from build123d import *

# Parameters (mm, degrees)
SKETCH1_R           = 16.5
BOSS_EXTRUDE1_DEPTH = 22
SKETCH2_W           = 2.99551857
SKETCH2_H           = 2.853303302
SKETCH2_W_2         = 2.853303302
SKETCH2_H_2         = 2.99551857
CUT_EXTRUDE1_DEPTH  = 2.5
SKETCH3_R           = 4
BOSS_EXTRUDE2_DEPTH = 2.2
CUT_EXTRUDE2_DEPTH  = 12.2
SKETCH5_W           = 3.219111416
SKETCH5_H           = 1.024262723
BOSS_EXTRUDE3_DEPTH = 3
CUT_EXTRUDE3_DEPTH  = 3
CIRPATTERN2_COUNT   = 2
SHELL1_START        = 2
SHELL1_DEPTH        = 20
SHELL1_START_2      = 14.2
SHELL1_2_DEPTH      = 7.8
SHELL1_START_3      = 4.5
SHELL1_3_DEPTH      = 9.7
SHELL1_START_4      = -0.2
SHELL1_4_OUTLINE_R  = 2
SHELL1_4_DEPTH      = 2.2
SKETCH7_R           = 9.780494134
CUT_EXTRUDE4_DEPTH  = 28
SKETCH8_R           = 16.5
SKETCH8_R_2         = 16.427034369
CUT_EXTRUDE5_DEPTH  = 0.3
FILLET1_R           = 0.3
FILLET2_R           = 0.8
SKETCH9_W           = 19.2
SKETCH9_H           = 1.567367832
SKETCH9_H_2         = 1.325546631
BOSS_EXTRUDE4_DEPTH = 3


# Read off the part's stored shape, not the designer's step: Shell1
with BuildPart() as part:
    # Sketch1 → Boss-Extrude1 (new body)
    with BuildSketch(Plane(origin=(0, 0, 0), x_dir=(0, 0, -1), z_dir=(1, 0, 0))):
        Circle(SKETCH1_R)
    extrude(amount=BOSS_EXTRUDE1_DEPTH)

    # Sketch2 → Cut-Extrude1 (cut)
    with BuildSketch(Plane.ZY):
        with Locations((-16.5, 0)):
            Rectangle(SKETCH2_W, SKETCH2_H)
        with Locations((0, 16.5)):
            Rectangle(SKETCH2_W_2, SKETCH2_H_2)
        with Locations((16.5, 0)):
            Rectangle(SKETCH2_W, SKETCH2_H)
        with Locations((0, -16.5)):
            Rectangle(SKETCH2_W_2, SKETCH2_H_2)
    extrude(amount=-CUT_EXTRUDE1_DEPTH, mode=Mode.SUBTRACT)

    # Sketch3 → Boss-Extrude2 (add)
    with BuildSketch(Plane.ZY):
        Circle(SKETCH3_R)
    extrude(amount=BOSS_EXTRUDE2_DEPTH)

    # Sketch4 → Cut-Extrude2 (cut)
    with BuildSketch(Plane.ZY):
        with BuildLine():
            ThreePointArc((2.706980055, 5.596864168), (0.036580812, 6.702979752), (-2.633818432, 5.596864168))
            ThreePointArc((-2.633818432, 5.596864168), (-2.633818432, 4.865247937), (-1.902202201, 4.865247937))
            ThreePointArc((-1.902202201, 4.865247937), (0.036580812, 5.668318155), (1.975363824, 4.865247937))
            ThreePointArc((1.975363824, 4.865247937), (2.706980055, 4.865247937), (2.706980055, 5.596864168))
        make_face()
        with BuildLine():
            ThreePointArc((-2.706980055, -5.596864168), (-0.036580812, -6.702979752), (2.633818432, -5.596864168))
            ThreePointArc((2.633818432, -5.596864168), (2.633818432, -4.865247937), (1.902202201, -4.865247937))
            ThreePointArc((1.902202201, -4.865247937), (-0.036580812, -5.668318155), (-1.975363824, -4.865247937))
            ThreePointArc((-1.975363824, -4.865247937), (-2.706980055, -4.865247937), (-2.706980055, -5.596864168))
        make_face()
    extrude(amount=-CUT_EXTRUDE2_DEPTH, mode=Mode.SUBTRACT)

    # Sketch5 → Boss-Extrude3 (add)
    with BuildSketch(Plane.ZY):
        with Locations((0, 11.230309148)):
            Rectangle(SKETCH5_W, SKETCH5_H)
    boss_extrude3 = extrude(amount=BOSS_EXTRUDE3_DEPTH)

    # Sketch6 → Cut-Extrude3 (cut)
    with BuildSketch(Plane(origin=(0, 11.742440509, 0), x_dir=(1, 0, 0), z_dir=(0, 1, 0))):
        with BuildLine():
            Line((-1.239883538, -0.443858464), (-2.275602474, -0.443858464))
            ThreePointArc((-2.275602474, -0.443858464), (-2.719460937, 0), (-2.275602474, 0.443858464))
            Line((-2.275602474, 0.443858464), (-1.239883538, 0.443858464))
            ThreePointArc((-1.239883538, 0.443858464), (-0.796025074, 0), (-1.239883538, -0.443858464))
        make_face()
    cut_extrude3 = extrude(amount=-CUT_EXTRUDE3_DEPTH, mode=Mode.SUBTRACT)

    # CirPattern2: Boss-Extrude3, Cut-Extrude3 ×2 about axis
    cirpattern2_axis = Axis((0, 0, 0), (1, 0, 0))
    add([boss_extrude3.rotate(cirpattern2_axis, i * 360 / CIRPATTERN2_COUNT) for i in range(1, CIRPATTERN2_COUNT)])
    add([cut_extrude3.rotate(cirpattern2_axis, i * 360 / CIRPATTERN2_COUNT) for i in range(1, CIRPATTERN2_COUNT)], mode=Mode.SUBTRACT)

    # Shell1 outline → Shell1 (cut)
    with BuildSketch(Plane.YZ.offset(SHELL1_START)):
        with BuildLine():
            Line((13.002240715, 3.426651651), (14.089288785, 3.426651651))
            ThreePointArc((14.089288785, 3.426651651), (10.253048327, 10.253048327), (3.426651651, 14.089288785))
            Line((3.426651651, 14.089288785), (3.426651651, 13.002240715))
            Line((3.426651651, 13.002240715), (-3.426651651, 13.002240715))
            Line((-3.426651651, 13.002240715), (-3.426651651, 14.089288785))
            ThreePointArc((-3.426651651, 14.089288785), (-10.253048327, 10.253048327), (-14.089288785, 3.426651651))
            Line((-14.089288785, 3.426651651), (-13.002240715, 3.426651651))
            Line((-13.002240715, 3.426651651), (-13.002240715, -3.426651651))
            Line((-13.002240715, -3.426651651), (-14.089288785, -3.426651651))
            ThreePointArc((-14.089288785, -3.426651651), (-10.253048327, -10.253048327), (-3.426651651, -14.089288785))
            Line((-3.426651651, -14.089288785), (-3.426651651, -13.002240715))
            Line((-3.426651651, -13.002240715), (3.426651651, -13.002240715))
            Line((3.426651651, -13.002240715), (3.426651651, -14.089288785))
            ThreePointArc((3.426651651, -14.089288785), (10.253048327, -10.253048327), (14.089288785, -3.426651651))
            Line((14.089288785, -3.426651651), (13.002240715, -3.426651651))
            Line((13.002240715, -3.426651651), (13.002240715, 3.426651651))
        make_face()
        with BuildLine():
            ThreePointArc((-3.451034375, 0.487988639), (-3.668318155, -0.036580811), (-3.451034375, -0.561150262))
            ThreePointArc((-3.451034375, -0.561150262), (-3.451034375, -4.121193617), (-7.01107773, -4.121193617))
            ThreePointArc((-7.01107773, -4.121193617), (-8.702979752, -0.036580811), (-7.01107773, 4.048031994))
            ThreePointArc((-7.01107773, 4.048031994), (-3.451034375, 4.048031994), (-3.451034375, 0.487988639))
        make_face(mode=Mode.SUBTRACT)
        with BuildLine():
            ThreePointArc((3.451034375, -0.487988639), (3.668318155, 0.036580811), (3.451034375, 0.561150262))
            ThreePointArc((3.451034375, 0.561150262), (3.451034375, 4.121193617), (7.01107773, 4.121193617))
            ThreePointArc((7.01107773, 4.121193617), (8.702979752, 0.036580811), (7.01107773, -4.048031994))
            ThreePointArc((7.01107773, -4.048031994), (3.451034375, -4.048031994), (3.451034375, -0.487988639))
        make_face(mode=Mode.SUBTRACT)
    extrude(amount=SHELL1_DEPTH, mode=Mode.SUBTRACT)

    # Shell1 2 outline → Shell1 2 (cut)
    with BuildSketch(Plane.YZ.offset(SHELL1_START_2)):
        with BuildLine():
            ThreePointArc((14.089288785, -3.426651651), (14.5, 0), (14.089288785, 3.426651651))
            Line((14.089288785, 3.426651651), (13.002240715, 3.426651651))
            Line((13.002240715, 3.426651651), (13.002240715, -3.426651651))
            Line((13.002240715, -3.426651651), (14.089288785, -3.426651651))
        make_face()
        with BuildLine():
            Line((3.426651651, 13.002240715), (3.426651651, 14.089288785))
            ThreePointArc((3.426651651, 14.089288785), (0, 14.5), (-3.426651651, 14.089288785))
            Line((-3.426651651, 14.089288785), (-3.426651651, 13.002240715))
            Line((-3.426651651, 13.002240715), (3.426651651, 13.002240715))
        make_face()
        with BuildLine():
            ThreePointArc((-3.426651651, -14.089288785), (0, -14.5), (3.426651651, -14.089288785))
            Line((3.426651651, -14.089288785), (3.426651651, -13.002240715))
            Line((3.426651651, -13.002240715), (-3.426651651, -13.002240715))
            Line((-3.426651651, -13.002240715), (-3.426651651, -14.089288785))
        make_face()
        with BuildLine():
            Line((-13.002240715, 3.426651651), (-14.089288785, 3.426651651))
            ThreePointArc((-14.089288785, 3.426651651), (-14.5, 0), (-14.089288785, -3.426651651))
            Line((-14.089288785, -3.426651651), (-13.002240715, -3.426651651))
            Line((-13.002240715, -3.426651651), (-13.002240715, 3.426651651))
        make_face()
        with BuildLine():
            ThreePointArc((-7.01107773, -4.121193617), (-3.451034375, -4.121193617), (-3.451034375, -0.561150262))
            ThreePointArc((-3.451034375, -0.561150262), (-3.668318155, -0.036580811), (-3.451034375, 0.487988639))
            ThreePointArc((-3.451034375, 0.487988639), (-3.451034375, 4.048031994), (-7.01107773, 4.048031994))
            ThreePointArc((-7.01107773, 4.048031994), (-8.702979752, -0.036580811), (-7.01107773, -4.121193617))
        make_face()
        with BuildLine():
            ThreePointArc((7.01107773, 4.121193617), (3.451034375, 4.121193617), (3.451034375, 0.561150262))
            ThreePointArc((3.451034375, 0.561150262), (3.668318155, 0.036580811), (3.451034375, -0.487988639))
            ThreePointArc((3.451034375, -0.487988639), (3.451034375, -4.048031994), (7.01107773, -4.048031994))
            ThreePointArc((7.01107773, -4.048031994), (8.702979752, 0.036580811), (7.01107773, 4.121193617))
        make_face()
    extrude(amount=SHELL1_2_DEPTH, mode=Mode.SUBTRACT)

    # Shell1 3 outline → Shell1 3 (cut)
    with BuildSketch(Plane.YZ.offset(SHELL1_START_3)):
        with BuildLine():
            ThreePointArc((14.089288785, -3.426651651), (14.5, 0), (14.089288785, 3.426651651))
            Line((14.089288785, 3.426651651), (13.002240715, 3.426651651))
            Line((13.002240715, 3.426651651), (13.002240715, -3.426651651))
            Line((13.002240715, -3.426651651), (14.089288785, -3.426651651))
        make_face()
        with BuildLine():
            Line((3.426651651, 13.002240715), (3.426651651, 14.089288785))
            ThreePointArc((3.426651651, 14.089288785), (0, 14.5), (-3.426651651, 14.089288785))
            Line((-3.426651651, 14.089288785), (-3.426651651, 13.002240715))
            Line((-3.426651651, 13.002240715), (3.426651651, 13.002240715))
        make_face()
        with BuildLine():
            ThreePointArc((-3.426651651, -14.089288785), (0, -14.5), (3.426651651, -14.089288785))
            Line((3.426651651, -14.089288785), (3.426651651, -13.002240715))
            Line((3.426651651, -13.002240715), (-3.426651651, -13.002240715))
            Line((-3.426651651, -13.002240715), (-3.426651651, -14.089288785))
        make_face()
        with BuildLine():
            Line((-13.002240715, 3.426651651), (-14.089288785, 3.426651651))
            ThreePointArc((-14.089288785, 3.426651651), (-14.5, 0), (-14.089288785, -3.426651651))
            Line((-14.089288785, -3.426651651), (-13.002240715, -3.426651651))
            Line((-13.002240715, -3.426651651), (-13.002240715, 3.426651651))
        make_face()
    extrude(amount=SHELL1_3_DEPTH, mode=Mode.SUBTRACT)

    # Shell1 4 outline → Shell1 4 (cut)
    with BuildSketch(Plane.YZ.offset(SHELL1_START_4)):
        Circle(SHELL1_4_OUTLINE_R)
    extrude(amount=SHELL1_4_DEPTH, mode=Mode.SUBTRACT)

    # Sketch7 → Cut-Extrude4 (cut)
    with BuildSketch(Plane(origin=(2, 0, 0), x_dir=(0, 0, -1), z_dir=(1, 0, 0))):
        Circle(SKETCH7_R)
    extrude(amount=CUT_EXTRUDE4_DEPTH, mode=Mode.SUBTRACT)

    # Sketch8 → Cut-Extrude5 (cut)
    with BuildSketch(Plane.ZY.offset(-2.5)):
        Circle(SKETCH8_R)
        Circle(SKETCH8_R_2, mode=Mode.SUBTRACT)
    extrude(amount=-CUT_EXTRUDE5_DEPTH, mode=Mode.SUBTRACT)

    # Fillet1
    fillet1_edges = [part.edges().sort_by_distance(p)[0] for p in [
        (0, 11.66726189, -11.66726189),
        (0, 11.66726189, 11.66726189),
        (0, -11.66726189, 11.66726189),
        (0, -11.66726189, -11.66726189),
    ]]
    fillet(fillet1_edges, radius=FILLET1_R)

    # Fillet2
    fillet2_edges = [part.edges().sort_by_distance(p)[0] for p in [
        (-3, 11.230309148, 1.609555708),
        (-3, 11.230309148, -1.609555708),
        (-3, -11.230309148, -1.609555708),
        (-3, -11.230309148, 1.609555708),
    ]]
    fillet(fillet2_edges, radius=FILLET2_R)

    # Sketch9 → Boss-Extrude4 (add)
    with BuildSketch(Plane.XY.offset(-14.58)):
        with Locations((12.4, 6.833683916)):
            Rectangle(SKETCH9_W, SKETCH9_H)
        with Locations((12.4, -6.712773316)):
            Rectangle(SKETCH9_W, SKETCH9_H_2)
    extrude(amount=-BOSS_EXTRUDE4_DEPTH)


solid = part.part
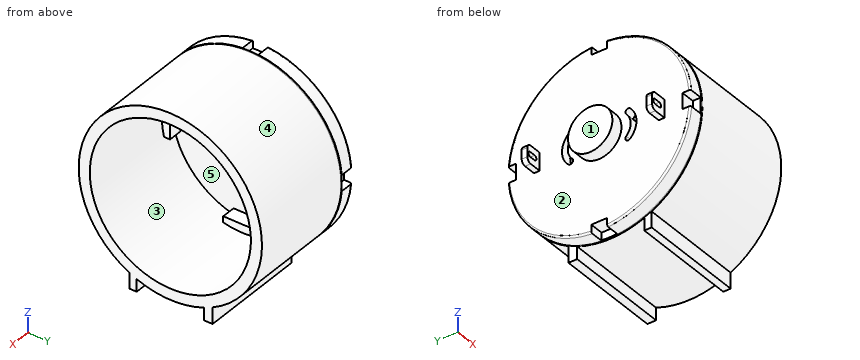
Geometry: final body of the model. Coordinates: model frame, mm. Face numbers are marked on the shaded views. A direction names the side the tool comes from. Round coordinates to 2 decimals unless told otherwise and drop trailing zeros. Order: outer loops, then holes, each group sorted by start corner. A loop starts at its lowest first (then second) coordinate and runs counter-clockwise, first axis right, second up.
Q1. Access query for the marked faces 1, 2 and 3. Directions: +Z, -Z, +X, -X, +Y, -Y. A direction counts if a zero-diameter tool reaches every point of the face in a straight line with its end or side. Return the directions, or none.
Result sheet:
face 1: +Z, -Z, -X
face 2: -X
face 3: +X
Q2. Pin query (flat end, axial travel): pin 1 (2 mm diameter, centred on x = 11, y = -4.5, fed in from -Z); pin 2 (0.8 mm diameter, centred on x = -1.5, y = 11.5, fed in from -Z); pin 3 (2 mm diameter, centred on y = 1, z = 0.5, fed in from +X). Return the tip coordinate at first contact, or that it passes through.
Result sheet:
pin 1: stops at z = -16.12
pin 2: stops at z = -1.61
pin 3: stops at x = 2
Q3. Section B-B, the plane y = 0. Output: boundary loops of the cut face in (x, z).
Result sheet:
outline: (-2.2, -4) - (0, -4) - (0, -15) - (2.5, -15) - (2.5, -16.43) - (2.8, -16.43) - (2.8, -16.5) - (22, -16.5) - (22, -14.5) - (4.5, -14.5) - (4.5, -13) - (2, -13) - (2, -2) - (-0.2, -2) - (-0.2, 2) - (2, 2) - (2, 13) - (4.5, 13) - (4.5, 14.5) - (22, 14.5) - (22, 16.5) - (2.8, 16.5) - (2.8, 16.43) - (2.5, 16.43) - (2.5, 15) - (0, 15) - (0, 4) - (-2.2, 4) - close
Q4. Mould query, pull axis Y, two halves, no side actions, for the marked faces 4 and 5. Classes: released by +Y, released by -Y, zero draft, split by the parting line, or undercut.
Result sheet:
face 4: split by the parting line
face 5: undercut
Q5. Material intervals for probe 1 along Z at (x, y) = (11, 0); probe 2 along Y at (x, z) = (1.5, 1), sorted ascending.
Result sheet:
probe 1: z = -16.5 to -14.5, 14.5 to 16.5
probe 2: y = -15 to -6.56, -5.46 to -1.73, 1.73 to 5.49, 6.58 to 15
Q6. Section C-C, the plane z = 0. Give the number of separate pieces and of enclosed holes in the cut face, and give its area (3 significant figures).
Result sheet:
separate pieces: 5
enclosed holes: 0
area: 153 mm2
Q7. Section A-A, the plane x = 8.5. Output: boundary loops of the cut face in (y, z), and give its area (3 significant figures).
Result sheet:
outline: (-7.38, -17.58) - (-6.05, -17.58) - (-6.05, -15.35) arc R16.5 ccw to (6.05, -15.35) - (6.05, -17.58) - (7.62, -17.58) - (7.62, -14.64) arc R16.5 ccw (long way) to (-7.38, -14.76) - close; hole circle Ø29 at (0, 0)
area: 202 mm2
